Check sheet for the modelled part. Datum: model origin and axes. Units: mm. Give positions to 0.01 mm unless a question says otherwise; leave off trailing zeros. Write each loop counter-clockwise with the first axis right and the second up, starting at its lowest first coordinate (ties: lowest second). Pieces come first, ordered by that corner, then holes. Notation, with made-up numbers: M -1,49 L 32,49 A18 cw 32,68 Z; hole C -20.5,80.25 d4. An arc over 180 degrees is marked long. Use CSV: the item, a comma, the result in double quotes. Start each with the question number.
1. Scan lines: line 1 (X direction, y = 1.85, z = 61.5); line 2 (X direction, y = 1.6, z = -20.5); line 3 (X direction, y = 0.7, z = -63). Record each from-to range of solid material in increasing order.
2. Cross-section at A-A, the plane x = -60. Enter the section's corners in (y, z), and give its area (3 significant figures).
3. Cross-section at B-B, the plane z = 1. Enter the section's corners in (x, y), and give its area (3 significant figures).
4. Cross-section at C-C, the plane y = 1.3. State how many separate pieces and enclosed holes the cut face has, and give its area (3 significant figures).
5. Depth check by flat-ended pin: P1, Ø0.6, axis at x = 103.5, y = 1, coming from the +Z side; P2, Ø1, axis at x = -22, y = 0.5, coming from the +Z side. Enter the tip coordinate at first touch or a pass-through.
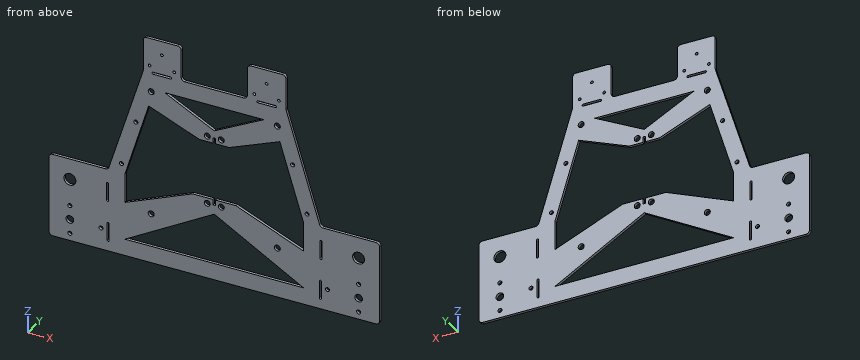
from build123d import *

# Parameters (mm, degrees)
SKETCH26_R          = 1
SKETCH26_R_2        = 2.15
SKETCH26_R_3        = 1.45
SKETCH26_R_4        = 4.25
SKETCH26_R_5        = 2.75
BOSS_EXTRUDE4_DEPTH = 2


with BuildPart() as part:
    # Sketch26 → Boss-Extrude4 (new body)
    with BuildSketch(Plane(origin=(0, 0, 0), x_dir=(1, 0, 0), z_dir=(0, 1, 0))):
        with BuildLine():
            Line((-20.877618357, -51.176455051), (21.352676296, -51.176455051))
            ThreePointArc((21.352676296, -51.176455051), (23.120443249, -51.908688098), (23.852676296, -53.676455051))
            Line((23.852676296, -53.676455051), (23.852676296, -73.676455051))
            ThreePointArc((23.852676296, -73.676455051), (24.584909343, -75.444222004), (26.352676296, -76.176455051))
            Line((26.352676296, -76.176455051), (48.872676296, -76.176455051))
            ThreePointArc((48.872676296, -76.176455051), (50.640443249, -75.444222004), (51.372676296, -73.676455051))
            Line((51.372676296, -73.676455051), (51.372676296, -51.552742091))
            ThreePointArc((51.372676296, -51.552742091), (51.400522432, -51.180646307), (51.483440514, -50.816839667))
            Line((51.483440514, -50.816839667), (75.469917209, 27.059447373))
            ThreePointArc((75.469917209, 27.059447373), (76.374187682, 28.334733163), (77.859152991, 28.823544949))
            Line((77.859152991, 28.823544949), (115.689249226, 28.823544949))
            ThreePointArc((115.689249226, 28.823544949), (117.457016179, 29.555777996), (118.189249226, 31.323544949))
            Line((118.189249226, 31.323544949), (118.189249226, 86.323544949))
            ThreePointArc((118.189249226, 86.323544949), (117.457016179, 88.091311902), (115.689249226, 88.823544949))
            Line((115.689249226, 88.823544949), (76.013272408, 88.823544949))
            Line((76.013272408, 88.823544949), (-75.538214468, 88.823544949))
            Line((-75.538214468, 88.823544949), (-76.032763958, 88.823544949))
            Line((-76.032763958, 88.823544949), (-115.214191287, 88.823544949))
            ThreePointArc((-115.214191287, 88.823544949), (-116.98195824, 88.091311902), (-117.714191287, 86.323544949))
            Line((-117.714191287, 86.323544949), (-117.714191287, 31.323544949))
            ThreePointArc((-117.714191287, 31.323544949), (-116.98195824, 29.555777996), (-115.214191287, 28.823544949))
            Line((-115.214191287, 28.823544949), (-77.373372177, 28.823544949))
            ThreePointArc((-77.373372177, 28.823544949), (-75.894006821, 28.338855879), (-74.98826724, 27.072727465))
            Line((-74.98826724, 27.072727465), (-50.52440331, -50.81067398))
            ThreePointArc((-50.52440331, -50.81067398), (-50.438398947, -51.180885745), (-50.409508246, -51.559856495))
            Line((-50.409508246, -51.559856495), (-50.409508246, -73.676455051))
            ThreePointArc((-50.409508246, -73.676455051), (-49.677275199, -75.444222004), (-47.909508246, -76.176455051))
            Line((-47.909508246, -76.176455051), (-25.877618357, -76.176455051))
            ThreePointArc((-25.877618357, -76.176455051), (-24.109851404, -75.444222004), (-23.377618357, -73.676455051))
            Line((-23.377618357, -73.676455051), (-23.377618357, -53.676455051))
            ThreePointArc((-23.377618357, -53.676455051), (-22.64538531, -51.908688098), (-20.877618357, -51.176455051))
        make_face()
        with Locations((-37.137618357, -66.176455051)):
            Circle(SKETCH26_R, mode=Mode.SUBTRACT)
        with Locations((-45.897618357, -56.176455051)):
            Circle(SKETCH26_R, mode=Mode.SUBTRACT)
        with Locations((-28.377618357, -56.176455051)):
            Circle(SKETCH26_R, mode=Mode.SUBTRACT)
        with BuildLine():
            Line((-43.378108588, -50.422722318), (-30.878108588, -50.422722318))
            ThreePointArc((-30.878108588, -50.422722318), (-30.128108588, -51.172722318), (-30.878108588, -51.922722318))
            Line((-30.878108588, -51.922722318), (-43.378108588, -51.922722318))
            ThreePointArc((-43.378108588, -51.922722318), (-44.128108588, -51.172722318), (-43.378108588, -50.422722318))
        make_face(mode=Mode.SUBTRACT)
        with Locations((-44.76247103, -37.176455051)):
            Circle(SKETCH26_R_2, mode=Mode.SUBTRACT)
        with Locations((-4.76247103, -15.676455051)):
            Circle(SKETCH26_R_2, mode=Mode.SUBTRACT)
        with Locations((-55.732763009, -11.697986619)):
            Circle(SKETCH26_R_3, mode=Mode.SUBTRACT)
        with Locations((28.852676296, -56.176455051)):
            Circle(SKETCH26_R, mode=Mode.SUBTRACT)
        with Locations((37.612676296, -66.176455051)):
            Circle(SKETCH26_R, mode=Mode.SUBTRACT)
        with Locations((46.372676296, -56.176455051)):
            Circle(SKETCH26_R, mode=Mode.SUBTRACT)
        with BuildLine():
            ThreePointArc((31.353166528, -51.922722318), (30.603166528, -51.172722318), (31.353166528, -50.422722318))
            Line((31.353166528, -50.422722318), (43.853166528, -50.422722318))
            ThreePointArc((43.853166528, -50.422722318), (44.603166528, -51.172722318), (43.853166528, -51.922722318))
            Line((43.853166528, -51.922722318), (31.353166528, -51.922722318))
        make_face(mode=Mode.SUBTRACT)
        with Locations((45.23752897, -37.176455051)):
            Circle(SKETCH26_R_2, mode=Mode.SUBTRACT)
        Polygon((35.658255702, -39.176455051), (-35.183197763, -39.176455051), (0.23752897, -20.965122509), align=None, mode=Mode.SUBTRACT)
        with Locations((5.23752897, -15.676455051)):
            Circle(SKETCH26_R_2, mode=Mode.SUBTRACT)
        with Locations((56.207820949, -11.697986619)):
            Circle(SKETCH26_R_3, mode=Mode.SUBTRACT)
        with Locations((-66.035396945, 21.75131433)):
            Circle(SKETCH26_R_3, mode=Mode.SUBTRACT)
        with Locations((-102.838214468, 43.823544949)):
            Circle(SKETCH26_R_4, mode=Mode.SUBTRACT)
        with BuildLine():
            ThreePointArc((-75.160005035, 39.191107079), (-75.910005035, 38.441107079), (-76.660005035, 39.191107079))
            Line((-76.660005035, 39.191107079), (-76.660005035, 51.691107079))
            ThreePointArc((-76.660005035, 51.691107079), (-75.910005035, 52.441107079), (-75.160005035, 51.691107079))
            Line((-75.160005035, 51.691107079), (-75.160005035, 39.191107079))
        make_face(mode=Mode.SUBTRACT)
        Polygon((-10.456903842, -11.676455051), (-46.597804641, -26.176455051), (-63.538214468, 28.823544949), (-63.538214468, 49.70968094), (-15.178445609, 29.823544949), (-0.76247103, 29.823544949), (-0.76247103, 33.823544949), (1.23752897, 33.823544949), (1.23752897, 29.823544949), (15.653503549, 29.823544949), (64.013272408, 49.70968094), (64.013272408, 28.823544949), (47.072862581, -26.176455051), (10.931961782, -11.676455051), (1.23752897, -11.676455051), (1.23752897, -15.676455051), (-0.76247103, -15.676455051), (-0.76247103, -11.676455051), align=None, mode=Mode.SUBTRACT)
        with Locations((-4.76247103, 33.823544949)):
            Circle(SKETCH26_R_2, mode=Mode.SUBTRACT)
        with Locations((-102.838214468, 63.123544949)):
            Circle(SKETCH26_R_3, mode=Mode.SUBTRACT)
        with Locations((-102.838214468, 73.323544949)):
            Circle(SKETCH26_R_5, mode=Mode.SUBTRACT)
        with Locations((-102.838214468, 83.523544949)):
            Circle(SKETCH26_R_3, mode=Mode.SUBTRACT)
        with Locations((-80.638214468, 73.323544949)):
            Circle(SKETCH26_R_3, mode=Mode.SUBTRACT)
        with BuildLine():
            ThreePointArc((-76.288214468, 81.095149015), (-75.538214468, 81.845149015), (-74.788214468, 81.095149015))
            Line((-74.788214468, 81.095149015), (-74.788214468, 68.595149015))
            ThreePointArc((-74.788214468, 68.595149015), (-75.538214468, 67.845149015), (-76.288214468, 68.595149015))
            Line((-76.288214468, 68.595149015), (-76.288214468, 81.095149015))
        make_face(mode=Mode.SUBTRACT)
        with Locations((-44.76247103, 52.823544949)):
            Circle(SKETCH26_R_2, mode=Mode.SUBTRACT)
        Polygon((0.23752897, 40.436613896), (-63.538214468, 76.823544949), (64.013272408, 76.823544949), align=None, mode=Mode.SUBTRACT)
        with Locations((5.23752897, 33.823544949)):
            Circle(SKETCH26_R_2, mode=Mode.SUBTRACT)
        with Locations((66.510454885, 21.75131433)):
            Circle(SKETCH26_R_3, mode=Mode.SUBTRACT)
        with BuildLine():
            Line((77.135062974, 51.691107079), (77.135062974, 39.191107079))
            ThreePointArc((77.135062974, 39.191107079), (76.385062974, 38.441107079), (75.635062974, 39.191107079))
            Line((75.635062974, 39.191107079), (75.635062974, 51.691107079))
            ThreePointArc((75.635062974, 51.691107079), (76.385062974, 52.441107079), (77.135062974, 51.691107079))
        make_face(mode=Mode.SUBTRACT)
        with Locations((103.313272408, 43.823544949)):
            Circle(SKETCH26_R_4, mode=Mode.SUBTRACT)
        with Locations((45.23752897, 52.823544949)):
            Circle(SKETCH26_R_2, mode=Mode.SUBTRACT)
        with Locations((103.313272408, 63.123544949)):
            Circle(SKETCH26_R_3, mode=Mode.SUBTRACT)
        with Locations((81.113272408, 73.323544949)):
            Circle(SKETCH26_R_3, mode=Mode.SUBTRACT)
        with BuildLine():
            Line((75.263272408, 68.595149015), (75.263272408, 81.095149015))
            ThreePointArc((75.263272408, 81.095149015), (76.013272408, 81.845149015), (76.763272408, 81.095149015))
            Line((76.763272408, 81.095149015), (76.763272408, 68.595149015))
            ThreePointArc((76.763272408, 68.595149015), (76.013272408, 67.845149015), (75.263272408, 68.595149015))
        make_face(mode=Mode.SUBTRACT)
        with Locations((103.313272408, 73.323544949)):
            Circle(SKETCH26_R_5, mode=Mode.SUBTRACT)
        with Locations((103.313272408, 83.523544949)):
            Circle(SKETCH26_R_3, mode=Mode.SUBTRACT)
    extrude(amount=BOSS_EXTRUDE4_DEPTH)


solid = part.part
Worked answers:
1,line 1,"x = -50.41 to -23.38, 23.85 to 51.37"
1,line 2,"x = -72.92 to -66.77, -65.3 to -60.97, 61.45 to 65.78, 67.24 to 73.45"
1,line 3,"x = -117.71 to -104.28, -101.39 to -39.31, 39.78 to 101.87, 104.76 to 118.19"
2,outline,"M 0,-88.82 L 2,-88.82 L 2,-76.82 L 0,-76.82 Z; M 0,-74.8 L 2,-74.8 L 2,-48.25 L 0,-48.25 Z; M 0,-17.34 L 2,-17.34 L 2,20.64 L 0,20.64 Z"
2,area,"153 mm^2"
3,outline,"M -66.17,0 L -54.35,0 L -54.35,2 L -66.17,2 Z; M 54.83,0 L 66.83,0 L 66.83,2 L 54.83,2 Z"
3,area,"47.6 mm^2"
4,separate pieces,"1"
4,enclosed holes,"37"
4,area,"15,800 mm^2"
5,P1,"stops at z = -28.82"
5,P2,"stops at z = 51.77"
